Check sheet for the modelled part. Datum: model origin and axes. Units: mm. Round coordinates to 2 decimals unless told otherwise and drop trailing zeros. Loops run counter-clockwise (first coordinate to the right, second up) from the corner with the lowest first, then second, coordinate; pieces in that order, holes last. Notation, with made-up numbers: (58.5, -29.5) - (64.5, -29.5) arc R7 ccw to (64.5, -25.5) - close; hole circle Ø3 at (-4, 22). An arc over 180 degrees is marked (long way). Return JSON: item names as keys, results as strings.
from build123d import *

# Parameters (mm, degrees)
F1_DEPTH = 3.7
F2_SIZE  = 1


with BuildPart() as f1:
    # F0 (on Right) → F1 (new body, symmetric)
    with BuildSketch(Plane.YZ):
        with BuildLine():
            Line((0, -9.8), (0, 0))
            Line((0, 0), (0, 5.650941))
            ThreePointArc((0, 5.650941), (-2.516585, 10.13472), (-3.4, 15.2))
            Line((-3.4, 15.2), (-4.9, 15.2))
            Line((-4.9, 15.2), (-4.9, -9.8))
            Line((-4.9, -9.8), (0, -9.8))
        make_face()
    extrude(amount=F1_DEPTH, both=True)

    # F2
    f2_edges = [f1.edges().sort_by_distance(p)[0] for p in [
        (0, -4.9, -9.8),
        (0, 0, -9.8),
        (3.7, -2.45, -9.8),
        (-3.7, -2.45, -9.8),
    ]]
    chamfer(f2_edges, length=F2_SIZE)


solid = f1.part
Q1. Sectioned sample at C-C (x = -3). Enter the section's corners in (y, z).
Answer key:
{"outline": "(-4.9, -8.8) - (-4.2, -9.5) - (-0.7, -9.5) - (0, -8.8) - (0, 5.65) arc R15.25 cw to (-3.4, 15.2) - (-4.9, 15.2) - close"}
Q2. Sectioned sample at A-A (x = 1.5). Enter the section's corners in (y, z).
Answer key:
{"outline": "(-4.9, -8.8) - (-3.9, -9.8) - (-1, -9.8) - (0, -8.8) - (0, 5.65) arc R15.25 cw to (-3.4, 15.2) - (-4.9, 15.2) - close"}
Q3. Sectioned sample at B-B (y = -4.3). Enter the section's corners in (x, z), plus the area to 3 significant figures.
Answer key:
{"outline": "(-3.7, -8.8) - (-3.1, -9.4) - (3.1, -9.4) - (3.7, -8.8) - (3.7, 15.2) - (-3.7, 15.2) - close", "area": "182 mm²"}
Q4. Scan lines: probe 1 along Z at (x, y) = (1.25, -4.2); probe 2 along Y at (x, z) = (-1.25, 10); probe 3 along Z at (x, y) = (-3.25, -1.85). Record each from-to range of solid material in increasing order. Write a range as [from, to].
Answer key:
{"probe 1": "z = [-9.5, 15.2]", "probe 2": "y = [-4.9, -2.47]", "probe 3": "z = [-9.25, 8.55]"}
Q5. Sectioned sample at D-D (z = 12.25). Enter the section's corners in (x, y).
Answer key:
{"outline": "(-3.7, -4.9) - (3.7, -4.9) - (3.7, -3.1) - (-3.7, -3.1) - close"}
